from build123d import *

# Parameters (mm, degrees)
SKETCH_1_R          = 1.1
EXTRUDE_1_DEPTH     = 13
EXTRUDE_2_DEPTH     = 4
CUT_EXTRUDE_1_DEPTH = 2
SKETCH_4_R          = 3.738204999
CUT_EXTRUDE_2_DEPTH = 2
EXTRUDE_4_DEPTH     = 7
CUT_EXTRUDE_START   = -10
SKETCH_9_R          = 3.75
CUT_EXTRUDE_3_DEPTH = 10
SKETCH_10_W         = 20
SKETCH_10_H         = 16
EXTRUDE_5_DEPTH     = 2.25
CHAMFER_1_SIZE      = 2.5
EXTRUDE_8_DEPTH     = 2
CUT_EXTRUDE_4_DEPTH = 1.25
SKETCH_11_R         = 3.6
EXTRUDE_9_DEPTH     = 5.25
SKETCH_15_W         = 17.5
SKETCH_15_H         = 14
EXTRUDE_10_DEPTH    = 1.25
CHAMFER_2_SIZE      = 12
CHAMFER_2_SIZE_2    = 8.402490459
CHAMFER_3_SIZE      = 8.402490459
CHAMFER_3_SIZE_2    = 12
CHAMFER_4_SIZE      = 2
CHAMFER_4_SIZE2     = 1.400415076


with BuildPart() as part:
    # 草图1 → 凸台-拉伸1 (new body)
    with BuildSketch(Plane.XY):
        Polygon((15, 16), (-15, 16), (-15, 32), (-19, 32), (-19, 0), (-11.784120735, 0), (-11.784120735, 13), (11.75, 13), (11.75, 0), (19, 0), (19, 32), (15, 32), align=None)
        with Locations(Location((-14, 6.5, 0), (0, 0, 180))):
            Circle(SKETCH_1_R, mode=Mode.SUBTRACT)
        with Locations(Location((14, 6.5, 0), (0, 0, 180))):
            Circle(SKETCH_1_R, mode=Mode.SUBTRACT)
    extrude(amount=EXTRUDE_1_DEPTH)

    # 草图2 → 凸台-拉伸2 (add)
    with BuildSketch(Plane(origin=(19, 0, 0), x_dir=(0, 0, -1), z_dir=(1, 0, 0))):
        with BuildLine():
            Line((0, 32), (-13, 32))
            ThreePointArc((-13, 32), (-6.5, 38.5), (0, 32))
        make_face()
    extrude_2 = extrude(amount=-EXTRUDE_2_DEPTH)

    # 镜向1: 凸台-拉伸2 across plane
    add(extrude_2.mirror(Plane(origin=(0, 0, 0), x_dir=(0, 0, 1), z_dir=(1, 0, 0))))

    # 草图3 → 切除-拉伸1 (cut)
    with BuildSketch(Plane.ZY.offset(19)):
        with BuildLine():
            Line((2.771151248, 31.602272727), (4.511280666, 15.287878788))
            ThreePointArc((4.511280666, 15.287878788), (6.5, 13.5), (8.488719334, 15.287878788))
            Line((8.488719334, 15.287878788), (10.228848752, 31.602272727))
            ThreePointArc((10.228848752, 31.602272727), (6.5, 35.75), (2.771151248, 31.602272727))
        make_face()
    extrude(amount=-CUT_EXTRUDE_1_DEPTH, mode=Mode.SUBTRACT)

    # 草图4 → 切除-拉伸2 (cut)
    with BuildSketch(Plane.ZY.offset(17)):
        with Locations((6.5, 32)):
            Circle(SKETCH_4_R)
    extrude(amount=-CUT_EXTRUDE_2_DEPTH, mode=Mode.SUBTRACT)

    # 草图5 → 凸台-拉伸4 (add)
    with BuildSketch(Plane(origin=(0, 0, 0), x_dir=(-1, 0, 0), z_dir=(0, 0, -1))):
        Polygon((-19, 16), (19, 16), (19, 0), (16.5, 0), (16.5, 14), (-16.5, 14), (-16.5, 0), (-19, 0), align=None)
    extrude(amount=EXTRUDE_4_DEPTH)

    # 草图9 → 切除-拉伸3 (cut)
    with BuildSketch(Plane(origin=(19, 0, 0), x_dir=(0, 0, -1), z_dir=(1, 0, 0)).offset(CUT_EXTRUDE_START)):
        with Locations(Location((-6.5, 32, 0), (0, 0, 90))):
            Circle(SKETCH_9_R)
    extrude(amount=CUT_EXTRUDE_3_DEPTH, mode=Mode.SUBTRACT)

    # 草图10 → 凸台-拉伸5 (add)
    with BuildSketch(Plane(origin=(0, 0, -7), x_dir=(-1, 0, 0), z_dir=(0, 0, -1))):
        with Locations((9, 8)):
            Rectangle(SKETCH_10_W, SKETCH_10_H)
    extrude(amount=EXTRUDE_5_DEPTH)

    # 倒角1
    chamfer_1_edges = [part.edges().sort_by_distance(p)[0] for p in [
        (19, 0, 3),
    ]]
    chamfer(chamfer_1_edges, length=CHAMFER_1_SIZE)

    # 草图12 → 凸台-拉伸8 (add)
    with BuildSketch(Plane.XZ):
        with BuildLine():
            Line((1, 13), (16.5, 13))
            ThreePointArc((16.5, 13), (12.241770088, -0.55746905), (1, -9.25))
            Line((1, -9.25), (-19, -9.25))
            Line((-19, -9.25), (-19, 13))
            Line((-19, 13), (1, 13))
        make_face()
    extrude(amount=EXTRUDE_8_DEPTH)

    # 草图13 → 切除-拉伸4 (cut)
    with BuildSketch(Plane(origin=(0, 0, -9.25), x_dir=(-1, 0, 0), z_dir=(0, 0, -1))):
        Polygon((19, -2), (19, 16), (-1, 16), (-1, 0), (-1, -2), align=None)
    extrude(amount=-CUT_EXTRUDE_4_DEPTH, mode=Mode.SUBTRACT)

    # 草图11 → 凸台-拉伸9 (add)
    with BuildSketch(Plane.XY.offset(-7)):
        with Locations((-5, 6.5)):
            Circle(SKETCH_11_R)
    extrude(amount=-EXTRUDE_9_DEPTH)

    # 草图15 → 凸台-拉伸10 (add)
    with BuildSketch(Plane.XY.offset(-7)):
        with Locations((-7.75, 7)):
            Rectangle(SKETCH_15_W, SKETCH_15_H)
    extrude(amount=EXTRUDE_10_DEPTH)

    # 倒角2
    # the kernel refuses this chamfer: 12, 8.402490459 mm, written as the material it adds along each edge
    with BuildSketch(Plane(origin=(-15, 16, 0), x_dir=(0, 0.9997533347641299, 0.022209674198457065), z_dir=(-1, 0, 0))) as chamfer_2_piece_1_section:
        Polygon((CHAMFER_2_SIZE * 0.999753334764, CHAMFER_2_SIZE * 0.0222096741985), (-CHAMFER_2_SIZE_2 * 0.0222096741972, CHAMFER_2_SIZE_2 * 0.999753334707), (0, 0), align=None)
    chamfer_2_piece_1 = extrude(amount=4, mode=Mode.PRIVATE)
    chamfer_2_piece_1 = split(chamfer_2_piece_1, bisect_by=Plane(origin=(-17, 20.095500367, -8), z_dir=(0, 0, 1)), keep=Keep.TOP, mode=Mode.PRIVATE)
    add(chamfer_2_piece_1)

    # 倒角3
    # the kernel refuses this chamfer: 12, 8.402490459 mm, written as the material it adds along each edge
    with BuildSketch(Plane(origin=(19, 16, 0), x_dir=(0, -0.045263737714020834, -0.9989750717851553), z_dir=(-1, 0, 0))) as chamfer_3_piece_1_section:
        Polygon((CHAMFER_3_SIZE * 0.998975071728, -CHAMFER_3_SIZE * 0.0452637377114), (-CHAMFER_3_SIZE_2 * 0.045263737714, -CHAMFER_3_SIZE_2 * 0.998975071785), (0, 0), align=None)
    chamfer_3_piece_1 = extrude(amount=4, mode=Mode.PRIVATE)
    chamfer_3_piece_1 = split(chamfer_3_piece_1, bisect_by=Plane(origin=(17, 20.095500367, -7), z_dir=(0, 0, 1)), keep=Keep.TOP, mode=Mode.PRIVATE)
    add(chamfer_3_piece_1)

    # 倒角4
    chamfer_4_edges = [part.edges().sort_by_distance(p)[0] for p in [
        (-19, -2, 2.5),
    ]]
    chamfer_4_side = [part.faces().sort_by_distance(p)[0] for p in [
        (-19, 13.42478673, 3.080992557),
    ]]
    chamfer(chamfer_4_edges, length=CHAMFER_4_SIZE, length2=CHAMFER_4_SIZE2, reference=chamfer_4_side[0])


solid = part.part
Read the model definition and answer for the solid it produces. Units are mm, in the model's axes. A direction names the side the tool comes from. Give positions to 0.01 mm unless a question says otherwise; leave off trailing zeros. Loops run counter-clockwise (first coordinate to the right, second up) from the corner with the lowest first, then second, coordinate; pieces in that order, holes last. Notation, with made-up numbers: (48.25, -24) -> (68.25, -24) arc R23 cw to (68.25, -10) -> close; hole circle Ø3 at (-25.5, -9.5). An arc over 180 degrees is marked (long way). Use a Markdown table: item, result.
Q1. Section B-B, the plane z = 6.5 is taken. Count the separate pieces of the cut face and the enclosed holes in it, then the cut area to 3 significant figures.
Solved:
| item | result |
|---|---|
| separate pieces | 3 |
| enclosed holes | 3 |
| area | 450 mm^2 |
Q2. Each of these flat-tipped pins is pushed along its axis until it touches: pin 1 (4.5 mm diameter, centred on x = -16, y = 31, fed in from -Z); pin 2 (8 mm diameter, centred on x = 3, z = 7, fed in from +Y); pin 3 (8 mm diameter, centred on x = -7.5, y = 24, fed in from +Z); pin 4 (1.4 mm diameter, centred on y = -1, z = -8.5, fed in from -X). Where does it stop, or does it pass through?
Solved:
| item | result |
|---|---|
| pin 1 | stops at z = 0 |
| pin 2 | stops at y = 16 |
| pin 3 | passes through |
| pin 4 | stops at x = -18.64 |
Q3. A tool of negligible diameter and unlimited length cuts with its end or side. For faces 1 (the face through (-11.784, 6, 6)), 2 (the face through (-18.01, 23.56, 3.63)), 3 (the face through (-2.5, 13.3, 0)), from which of +Z, -Z, +X, -X, +Y, -Y can it reach the whole face along a straight path? Write none if from no direction.
Solved:
| item | result |
|---|---|
| face 1 | +Z |
| face 2 | -X |
| face 3 | none |
Q4. Determine the mould class of faces 4 (the face through (-12.9, 6.5, 6.4)), 5 (the face through (17, 38.5, 6.6)), 6 (the face through (-18.01, 35.75, 6.59)) for opening direction Z: pulls with the +Z half, pulls with the -Z half, needs draft (parallel to the pull), parting line crosses it, or undercut.
Solved:
| item | result |
|---|---|
| face 4 | needs draft |
| face 5 | parting line crosses it |
| face 6 | undercut |
Q5. Find the intervals of material crossed by line 1 along X through (y, z) = (6.5, 8.25); line 2 along X through (y, z) = (13.5, -0.5); line 3 along Z through (x, y) = (18.1, 32), in increasing order.
Solved:
| item | result |
|---|---|
| line 1 | x = -19 to -15.1, -12.9 to -11.78, 11.75 to 12.9, 15.1 to 19 |
| line 2 | x = -19 to -16.5, 16.5 to 19 |
| line 3 | z = 0 to 2.75, 10.25 to 13 |
Q6. Section A-A, the plane y = 6.5 is taken. Determine the outline of the cut face in (x, z).
Solved:
| item | result |
|---|---|
| outline | (-19, -8) -> (-8.6, -8) -> (-8.6, -12.25) -> (-1.4, -12.25) -> (-1.4, -8) -> (1, -8) -> (1, -5.75) -> (-16.5, -5.75) -> (-16.5, 0) -> (-15.1, 0) -> (-15.1, 13) -> (-19, 13) -> close; (-12.9, 0) -> (-11.78, 0) -> (-11.78, 13) -> (-12.9, 13) -> close; (11.75, 0) -> (12.9, 0) -> (12.9, 13) -> (11.75, 13) -> close; (15.1, 0) -> (16.5, 0) -> (16.5, -7) -> (19, -7) -> (19, 13) -> (15.1, 13) -> close |
Q7. Section C-C, the plane x = -14 is taken. Determine the outline of the cut face in (y, z), then the cut area to 3 significant figures.
Solved:
| item | result |
|---|---|
| outline | (-2, -8) -> (16, -8) -> (16, 13) -> (7.6, 13) -> (7.6, 0) -> (14, 0) -> (14, -5.75) -> (0, -5.75) -> (0, 0) -> (5.4, 0) -> (5.4, 13) -> (-2, 13) -> close |
| area | 269 mm^2 |
Q8. Section D-D, the plane y = 22.5 is taken. Determine the outline of the cut face in (x, z), then the cut area to 3 significant figures.
Solved:
| item | result |
|---|---|
| outline | (-19, -3.85) -> (-15, -3.85) -> (-15, 13) -> (-19, 13) -> (-19, 9.26) -> (-17, 9.26) -> (-17, 3.74) -> (-19, 3.74) -> close; (15, -3.85) -> (19, -3.85) -> (19, 13) -> (15, 13) -> close |
| area | 124 mm^2 |
